For this review, use the dimensioned drawing (mm, ordinates from the lowest corner) and the shaded views. Round coordinates to 2 decimals unless told otherwise and drop trailing zeros. Loops run counter-clockwise (first coordinate to the right, second up) from the corner with the lowest first, then second, coordinate; pieces in that order, holes last. Notation, with made-up numbers: (-29, 0.25) - (25, 0.25) arc R19 cw to (25, 26.25) - close; hole circle Ø9 at (75.5, 8.5). An arc over 180 degrees is marked (long way). Use one line per item in the form item = value. Start each with the question number.
(1) We need section A-A, the plane x = 123. Write out the cut boundary in (y, z), then the cut area to 3 significant figures.
(2) We need section B-B, the plane z = 11.75. Write out the cut boundary in (x, y).
(3) For pin 1 (1.2 mm diameter, centred on y = 6, z = 5.5, fed in from -X), flat-tipped, find the tip position at first contact; note if it passes through.
(4) Wall thickness on probe 1 along Z at (x, y) = (138, 9.5); probe 2 along X at (y, z) = (7.5, 17.5); probe 3 along Y at (x, z) = (22, 23.6): over which ranges is each line inside the solid? List them lowest first. Write a range as [from, to].
(5) We need section C-C, the plane y = 8.5. Give the number of separate pieces and of enclosed holes in the cut face, then the cut area to 3 significant figures.
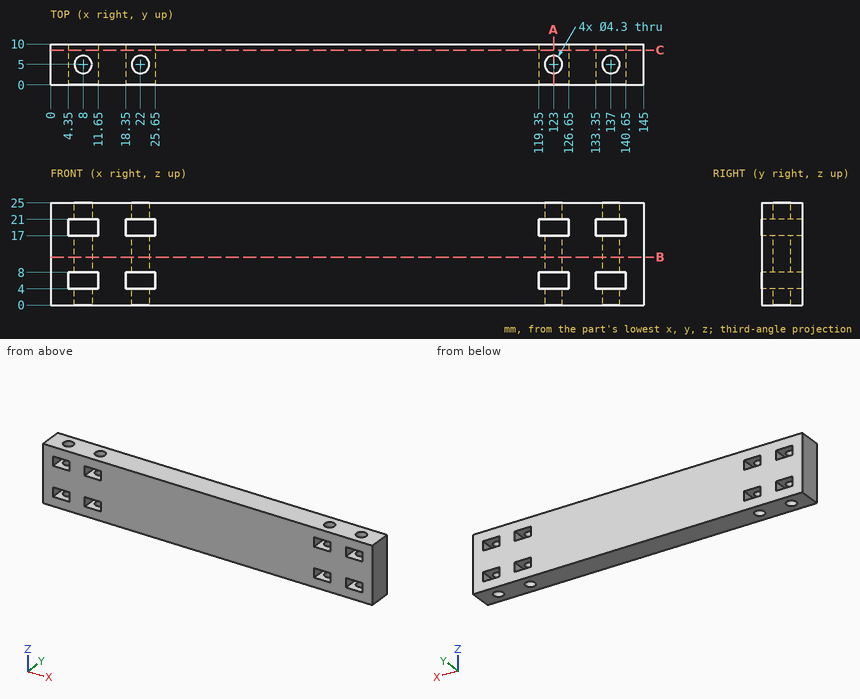
Data:
q1.outline = (0, 0) - (2.85, 0) - (2.85, 4) - (0, 4) - close; (0, 8) - (2.85, 8) - (2.85, 17) - (0, 17) - close; (0, 21) - (2.85, 21) - (2.85, 25) - (0, 25) - close; (7.15, 0) - (10, 0) - (10, 4) - (7.15, 4) - close; (7.15, 8) - (10, 8) - (10, 17) - (7.15, 17) - close; (7.15, 21) - (10, 21) - (10, 25) - (7.15, 25) - close
q1.area = 96.9 mm^2
q2.outline = (0, 0) - (145, 0) - (145, 10) - (0, 10) - close; hole circle Ø4.3 at (8, 5); hole circle Ø4.3 at (22, 5); hole circle Ø4.3 at (123, 5); hole circle Ø4.3 at (137, 5)
q3.pin_1 = 0
q4.probe_1 = [0, 4], [8, 17], [21, 25]
q4.probe_2 = [0, 4.35], [11.65, 18.35], [25.65, 119.35], [126.65, 133.35], [140.65, 145]
q4.probe_3 = [0, 2.85], [7.15, 10]
q5.separate_pieces = 1
q5.enclosed_holes = 8
q5.area = 3,390 mm^2
